```python
from build123d import *

# Parameters (mm, degrees)
SKETCH1_W           = 26
SKETCH1_H           = 32
SKETCH1_R           = 4.1021
BOSS_EXTRUDE1_DEPTH = 3
FILLET1_R           = 8
FILLET2_R           = 2


with BuildPart() as part:
    # Sketch1 → Boss-Extrude1 (new body)
    with BuildSketch(Plane.XY):
        with Locations((2, 0)):
            Rectangle(SKETCH1_W, SKETCH1_H)
        Circle(SKETCH1_R, mode=Mode.SUBTRACT)
    extrude(amount=BOSS_EXTRUDE1_DEPTH)

    # Fillet1
    fillet1_edges = [part.edges().sort_by_distance(p)[0] for p in [
        (15, -16, 1.5),
        (-11, -16, 1.5),
        (-11, 16, 1.5),
        (15, 16, 1.5),
    ]]
    fillet(fillet1_edges, radius=FILLET1_R)

    # Fillet2
    fillet2_edges = [part.edges().sort_by_distance(p)[0] for p in [
        (15, 0, 0),
        (2, -16, 0),
        (-11, 0, 0),
        (2, 16, 0),
        (-8.656854249, 13.656854249, 0),
        (12.656854249, 13.656854249, 0),
        (-8.656854249, -13.656854249, 0),
        (12.656854249, -13.656854249, 0),
    ]]
    fillet(fillet2_edges, radius=FILLET2_R)


solid = part.part
```
The listing builds one solid part. Answer for the finished solid, in the listing's coordinates (mm). Round coordinates to 2 decimals unless told otherwise and drop trailing zeros. Loops run counter-clockwise (first coordinate to the right, second up) from the corner with the lowest first, then second, coordinate; pieces in that order, holes last. Notation, with made-up numbers: (-11.5, 45) -> (27.5, 45) arc R30 cw to (27.5, 74) -> close; hole circle Ø2 at (-1.75, 68.25). An arc over 180 degrees is marked (long way). Use one line per item in the form item = value.
1. The part is cut by section B-B on y = 0. Determine the outline of the cut face in (x, z).
Answer key:
outline = (-11, 2) arc R2 ccw to (-9, 0) -> (-4.1, 0) -> (-4.1, 3) -> (-11, 3) -> close; (4.1, 0) -> (13, 0) arc R2 ccw to (15, 2) -> (15, 3) -> (4.1, 3) -> close
2. Flat-ended cylindrical pins translate along their axes: pin 1 Ø1 at (y, z) = (11, 2.5) entering from -X; pin 2 Ø5 at (x, y) = (0, 0) entering from -Z; pin 3 Ø1.5 at (x, z) = (8.5, 2) entering from -Y. Find the tip coordinate at first contact, or state that the pin passes through.
Answer key:
pin_1 = -10.6
pin_2 = through
pin_3 = -15.96
3. The part is cut by section A-A on x = 0. Determine the outline of the cut face in (y, z).
Answer key:
outline = (-16, 2) arc R2 ccw to (-14, 0) -> (-4.1, 0) -> (-4.1, 3) -> (-16, 3) -> close; (4.1, 0) -> (14, 0) arc R2 ccw to (16, 2) -> (16, 3) -> (4.1, 3) -> close
4. The part is cut by section D-D on x = 5.25. Determine the outline of the cut face in (y, z).
Answer key:
outline = (-16, 2) arc R2 ccw to (-14, 0) -> (14, 0) arc R2 ccw to (16, 2) -> (16, 3) -> (-16, 3) -> close
5. Find the intervals of material crossed by probe 1 along Y at (x, z) = (0.5, 2); probe 2 along X at (y, z) = (1, 1.6); probe 3 along Y at (x, z) = (0, 1), in increasing order. Write a range as [from, to].
Answer key:
probe_1 = [-16, -4.07], [4.07, 16]
probe_2 = [-10.96, -3.98], [3.98, 14.96]
probe_3 = [-15.73, -4.1], [4.1, 15.73]
6. For a pull along X with two mould halves and no side action, classify faces 1 (the cylindrical face through (-0.889, -4.005, 1.479)), 2 (the cylindrical face through (-10.4, -0.11, 0.57)), 3 (the cylindrical face through (14.4, 0.11, 0.57)) as released by +X, released by -X, zero draft, split by the parting line, or undercut.
Answer key:
face_1 = undercut
face_2 = released by -X
face_3 = released by +X
7. The part is cut by section C-C on y = 5. Determine the outline of the cut face in (x, z).
Answer key:
outline = (-11, 2) arc R2 ccw to (-9, 0) -> (13, 0) arc R2 ccw to (15, 2) -> (15, 3) -> (-11, 3) -> close
